Geometry check sheet. Reference: the model listing, model coordinates, mm. Round coordinates to 2 decimals unless told otherwise and drop trailing zeros. Write each loop counter-clockwise with the first axis right and the second up, starting at its lowest first coordinate (ties: lowest second). Pieces come first, ordered by that corner, then holes. Notation, with made-up numbers: M -36,21.25 L -32,21.25 A34 cw -32,57.25 Z; hole C 53,9 d10. An arc over 180 degrees is marked long. One line per item, written item: value. Start each with the question number.
1. Scan lines: probe 1 along X at (y, z) = (19, -3.75); probe 2 along Y at (x, z) = (0, -1.55); probe 3 along Z at (x, y) = (191, -12). Record each from-to range of solid material in increasing order. Write a range as [from, to].
2. Section check B-B (y = 0). Count the separate pieces of the cut face and the enclosed holes in it, and give its area (3 significant figures).
3. Section check D-D (y = 25). Record the boundary of the cut face in (x, z).
4. Depth check by flat-ended pin: P1, Ø7, axis at x = 14.94, y = -8.63, coming from the -Z side; P2, Ø6, axis at y = 11, z = -10, coming from the -X side. Enter the tip coordinate at first touch or a pass-through.
5. Section check A-A (x = 197). Record the boundary of the cut face in (y, z).
from build123d import *

# Parameters (mm, degrees)
BOSS_EXTRUDE2_DEPTH = 12
SKETCH2_R           = 2
CUT_EXTRUDE1_DEPTH  = 12
CIRPATTERN1_COUNT   = 6
SKETCH4_R           = 2
CUT_EXTRUDE2_DEPTH  = 12
CIRPATTERN2_COUNT   = 6
CUT_EXTRUDE4_DEPTH  = 12
SKETCH8_R           = 10
CUT_EXTRUDE5_DEPTH  = 12
SKETCH9_R           = 10
CUT_EXTRUDE6_DEPTH  = 12
SKETCH10_R          = 3.75
CUT_EXTRUDE7_DEPTH  = 6
CIRPATTERN3_COUNT   = 6
SKETCH11_R          = 3.75
CUT_EXTRUDE8_DEPTH  = 6
CIRPATTERN4_COUNT   = 6


with BuildPart() as part:
    # Sketch1 → Boss-Extrude2 (new body)
    with BuildSketch(Plane.XY):
        with BuildLine():
            Line((0, 29.5), (204.48, 29.5))
            ThreePointArc((204.48, 29.5), (233.98, 0), (204.48, -29.5))
            Line((204.48, -29.5), (0, -29.5))
            ThreePointArc((0, -29.5), (-29.5, 0), (0, 29.5))
        make_face()
    extrude(amount=-BOSS_EXTRUDE2_DEPTH)

    # Sketch2 → Cut-Extrude1 (cut)
    with BuildSketch(Plane.XY):
        with Locations((0, 17.25)):
            Circle(SKETCH2_R)
    cut_extrude1 = extrude(amount=-CUT_EXTRUDE1_DEPTH, mode=Mode.SUBTRACT)

    # CirPattern1: Cut-Extrude1 ×6 about axis
    cirpattern1_axis = Axis((0, 0, 0), (0, 0, 1))
    for i in range(1, CIRPATTERN1_COUNT):
        add(cut_extrude1.rotate(cirpattern1_axis, i * 360 / CIRPATTERN1_COUNT), mode=Mode.SUBTRACT)

    # Sketch4 → Cut-Extrude2 (cut)
    with BuildSketch(Plane.XY):
        with Locations((204.48, 17.25)):
            Circle(SKETCH4_R)
    cut_extrude2 = extrude(amount=-CUT_EXTRUDE2_DEPTH, mode=Mode.SUBTRACT)

    # CirPattern2: Cut-Extrude2 ×6 about axis
    cirpattern2_axis = Axis((204.48, 0, 0), (0, 0, 1))
    for i in range(1, CIRPATTERN2_COUNT):
        add(cut_extrude2.rotate(cirpattern2_axis, i * 360 / CIRPATTERN2_COUNT), mode=Mode.SUBTRACT)

    # Sketch7 → Cut-Extrude4 (cut)
    with BuildSketch(Plane.XY):
        with BuildLine():
            Line((56.938938215, -17.5), (36.938938215, 17.5))
            ThreePointArc((36.938938215, 17.5), (31.282083966, 15.156854249), (28.938938215, 9.5))
            Line((28.938938215, 9.5), (28.938938215, -9.5))
            ThreePointArc((28.938938215, -9.5), (31.282083966, -15.156854249), (36.938938215, -17.5))
            Line((36.938938215, -17.5), (56.938938215, -17.5))
        make_face()
        Polygon((88.938938215, 17.5), (48.938938215, 17.5), (68.938938215, -17.5), align=None)
        Polygon((120.938938215, -17.5), (100.938938215, 17.5), (80.938938215, -17.5), align=None)
        Polygon((152.938938215, 17.5), (112.938938215, 17.5), (132.938938215, -17.5), align=None)
        with BuildLine():
            Line((167.541061785, 17.5), (164.938938215, 17.5))
            Line((164.938938215, 17.5), (144.938938215, -17.5))
            Line((144.938938215, -17.5), (167.541061785, -17.5))
            ThreePointArc((167.541061785, -17.5), (173.197916034, -15.156854249), (175.541061785, -9.5))
            Line((175.541061785, -9.5), (175.541061785, 9.5))
            ThreePointArc((175.541061785, 9.5), (173.197916034, 15.156854249), (167.541061785, 17.5))
        make_face()
    extrude(amount=-CUT_EXTRUDE4_DEPTH, mode=Mode.SUBTRACT)

    # Sketch8 → Cut-Extrude5 (cut)
    with BuildSketch(Plane.XY):
        Circle(SKETCH8_R)
    extrude(amount=-CUT_EXTRUDE5_DEPTH, mode=Mode.SUBTRACT)

    # Sketch9 → Cut-Extrude6 (cut)
    with BuildSketch(Plane.XY):
        with Locations((204.48, 0)):
            Circle(SKETCH9_R)
    extrude(amount=-CUT_EXTRUDE6_DEPTH, mode=Mode.SUBTRACT)

    # Sketch10 → Cut-Extrude7 (cut)
    with BuildSketch(Plane(origin=(0, 0, -12), x_dir=(-1, 0, 0), z_dir=(0, 0, -1))):
        with Locations((-204.48, 17.25)):
            Circle(SKETCH10_R)
    cut_extrude7 = extrude(amount=-CUT_EXTRUDE7_DEPTH, mode=Mode.SUBTRACT)

    # CirPattern3: Cut-Extrude7 ×6 about axis
    cirpattern3_axis = Axis((204.48, 0, 0), (0, 0, 1))
    for i in range(1, CIRPATTERN3_COUNT):
        add(cut_extrude7.rotate(cirpattern3_axis, i * 360 / CIRPATTERN3_COUNT), mode=Mode.SUBTRACT)

    # Sketch11 → Cut-Extrude8 (cut)
    with BuildSketch(Plane(origin=(0, 0, -12), x_dir=(-1, 0, 0), z_dir=(0, 0, -1))):
        with Locations((0, 17.25)):
            Circle(SKETCH11_R)
    cut_extrude8 = extrude(amount=-CUT_EXTRUDE8_DEPTH, mode=Mode.SUBTRACT)

    # CirPattern4: Cut-Extrude8 ×6 about axis
    cirpattern4_axis = Axis((0, 0, 0), (0, 0, 1))
    for i in range(1, CIRPATTERN4_COUNT):
        add(cut_extrude8.rotate(cirpattern4_axis, i * 360 / CIRPATTERN4_COUNT), mode=Mode.SUBTRACT)


solid = part.part
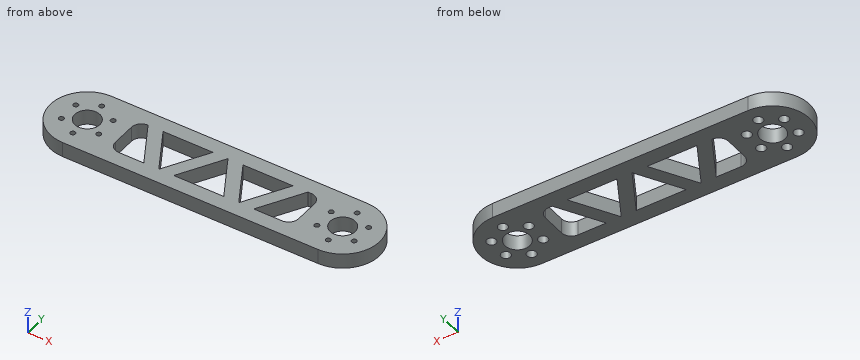
Result sheet:
1. probe 1: x = [-22.57, -0.97], [0.97, 203.51], [205.45, 227.05]
1. probe 2: y = [-29.5, -19.25], [-15.25, -10], [10, 15.25], [19.25, 29.5]
1. probe 3: z = [-6, 0]
2. separate pieces: 8
2. enclosed holes: 0
2. area: 1,500 mm2
3. outline: M -15.66,-12 L 220.14,-12 L 220.14,0 L -15.66,0 Z
4. P1: stops at z = -6
4. P2: stops at x = -28.39
5. outline: M -29.5,-12 L -6.64,-12 L -6.64,0 L -29.5,0 Z; M 6.64,-12 L 29.5,-12 L 29.5,0 L 6.64,0 Z
